Verification items for the finished model (mm, model axes). A direction names the side the tool comes from. Round coordinates to 2 decimals unless told otherwise and drop trailing zeros. Order: outer loops, then holes, each group sorted by start corner. A loop starts at its lowest first (then second) coordinate and runs counter-clockwise, first axis right, second up.
Autodesk Inventor part; units mm, degrees
ref_plane "YZ Plane" through (0, 0, 0) normal (1, 0, 0) x (0, 1, 0)
ref_plane "XZ Plane" through (0, 0, 0) normal (0, 1, 0) x (-1, 0, 0)
ref_plane "XY Plane" through (0, 0, 0) normal (0, 0, 1) x (1, 0, 0)
sketch "Sketch1" plane through (0, 0, 0) normal (0, 0, 1) x (1, 0, 0)
  line L0 (-41.2246, 0) -> (41.2246, 0)
  line L1 (-26.3201, 48.95) -> (26.3201, 48.95)
  circle A0 centre (-20, 36) radius 9.45
  line L2 (0, 48.95) -> (0, 0) construction
  circle A1 centre (-20, 36) radius 5
  circle A2 centre (20, 36) radius 9.45
  circle A3 centre (20, 36) radius 5
  arc A4 (-44.9834, 5.3681) -> (-41.2246, 0) centre (-41.2246, 4) ccw
  arc A5 (-26.3201, 48.95) -> (-30.0788, 46.3181) centre (-26.3201, 44.95) ccw
  line L3 (-44.9834, 5.3681) -> (-30.0788, 46.3181)
  arc A6 (41.2246, 0) -> (44.9834, 5.3681) centre (41.2246, 4) ccw
  arc A7 (30.0788, 46.3181) -> (26.3201, 48.95) centre (26.3201, 44.95) ccw
  line L4 (44.9834, 5.3681) -> (30.0788, 46.3181)
  dimension "d1" = 18.9
  dimension "d3" = 3.5
  dimension "d4" = 36
  dimension "d7" = 10
  dimension "d8" = 40
  dimension "d10" = 4
  dimension "d11" = 13
  dimension "d12" = 70
extrude "Extrusion1" add sketch "Sketch1" along normal mid plane 30 contours A4 L3 A5 L1 A7 L4 A6 L0
extrude "Extrusion2" add sketch "Sketch1" along normal mid plane 18 contours A0 | A2
properties part number "EngineMount"
1) Scan lines: probe 1 along X at (y, z) = (29, 9.5); probe 2 along Y at (x, z) = (-20, 11.3); probe 3 along X at (y, z) = (44, 11.5). Record each from-to range of solid material in increasing order.
2) Sectioned sample at C-C on y = 36. Record the cut outline in (x, z), then the cut area to 3 significant figures.
3) Sectioned sample at B-B on x = 20. Record the cut outline in (y, z), then the cut area to 3 significant figures.
4) Tool access check on faces 5 (the flat face through (-16, 32, -9)), 6 (the flat face through (-16, 32, 9)), 7 (the flat face through (37.635, 25.556, -0.21)). Record the directions out of +Z, -Z, +X, -X, +Y, -Y that give a thin tool (end or side, any length) a straight path to the whole face; none if there is none.
5) Sectioned sample at D-D on x = -13.5. Record the cut outline in (y, z), then the cut area to 3 significant figures.
6) Go/stop test with flat-tipped pins: pin 1 Ø10 at (x, z) = (2.5, -8.5) entering from -Y; pin 2 Ø9.5 at (x, y) = (-20.5, 38) entering from -Z; pin 3 Ø11.5 at (x, y) = (20, 36) entering from +Z; pin 4 Ø5 at (y, z) = (30.5, 6.5) entering from +X. Record where each tip stops, or that it passes through.
7) Sectioned sample at A-A on z = 7.75. Record the cut outline in (x, y).
8) Draft check along X on faces 1 (the cylindrical face through (18.77, 26.63, 11.96)), 2 (the cylindrical face through (28.586, 48.246, -0.21)), 3 (the flat face through (0, 48.95, 0)), 4 (the cylindrical face through (-44.47, 1.66, -0.21)). Enter one of: released by +X, released by -X, zero draft, split by the parting line, or undercut.
Returned:
1. probe 1: x = -36.38 to -26.35, -13.65 to 13.65, 26.35 to 36.38
1. probe 2: y = 0 to 26.55, 45.45 to 48.95
1. probe 3: x = -30.92 to -25.03, -14.97 to 14.97, 25.03 to 30.92
2. outline: (-33.83, -15) - (-29.45, -15) - (-29.45, -9) - (-25, -9) - (-25, 9) - (-29.45, 9) - (-29.45, 15) - (-33.83, 15) - close; (-15, -9) - (-10.55, -9) - (-10.55, -15) - (10.55, -15) - (10.55, -9) - (15, -9) - (15, 9) - (10.55, 9) - (10.55, 15) - (-10.55, 15) - (-10.55, 9) - (-15, 9) - close; (25, -9) - (29.45, -9) - (29.45, -15) - (33.83, -15) - (33.83, 15) - (29.45, 15) - (29.45, 9) - (25, 9) - close
2. area: 1,220 mm2
3. outline: (0, -15) - (26.55, -15) - (26.55, -9) - (31, -9) - (31, 9) - (26.55, 9) - (26.55, 15) - (0, 15) - close; (41, -9) - (45.45, -9) - (45.45, -15) - (48.95, -15) - (48.95, 15) - (45.45, 15) - (45.45, 9) - (41, 9) - close
3. area: 1,060 mm2
4. face 5: -Z
4. face 6: +Z
4. face 7: +Z, -Z, +X, +Y
5. outline: (0, -15) - (29.14, -15) - (29.14, -9) - (42.86, -9) - (42.86, -15) - (48.95, -15) - (48.95, 15) - (42.86, 15) - (42.86, 9) - (29.14, 9) - (29.14, 15) - (0, 15) - close
5. area: 1,300 mm2
6. pin 1: stops at y = 0
6. pin 2: stops at z = -9
6. pin 3: stops at z = 9
6. pin 4: stops at x = 36.75
7. outline: (-44.98, 5.37) arc R4 ccw to (-41.22, 0) - (41.22, 0) arc R4 ccw to (44.98, 5.37) - (30.08, 46.32) arc R4 ccw to (26.32, 48.95) - (-26.32, 48.95) arc R4 ccw to (-30.08, 46.32) - close; hole circle Ø10 at (-20, 36); hole circle Ø10 at (20, 36)
8. face 1: undercut
8. face 2: released by +X
8. face 3: zero draft
8. face 4: released by -X
